Verification items for the finished model (mm, model axes). Face numbers are marked on the shaded views. A direction names the side the tool comes from. Give positions to 0.01 mm unless a question says otherwise; leave off trailing zeros. Order: outer loops, then holes, each group sorted by start corner. A loop starts at its lowest first (then second) coordinate and runs counter-clockwise, first axis right, second up. Notation, with made-up numbers: (49.25, 34) - (86.25, 34) arc R22 ccw to (86.25, 62) - close; hole circle Ø6 at (-5, -32). An arc over 180 degrees is marked (long way). Answer as a JSON object with one key per item and string values. Group by question number.
(1) Thickness scan on line 1 (X direction, y = 1.95, z = 0); line 2 (X direction, y = 5.5, z = 0); line 3 (Y direction, x = -5, z = 2.25). Record the ranges inside material, lowest first.
(2) Mould release check, pull along Z, two halves, no side actions. Record for the marked faces 6, 7 and 8: +Z half, -Z half, draft (parallel to the pull), parting line (faces both ways), or undercut.
(3) Access from +Z, -Z, +X, -X, +Y, -Y to the whole of each face (thin tool, end or side, straight path). Record for the marked faces 1, 2, 3, 4 and 5.
(4) Section check B-B (y = 5.75). Record the boundary of the cut face in (x, z).
(5) Section check C-C (z = 0.75). Record the boundary of the cut face in (x, y), then the cut area to 3 significant figures.
(6) Section check A-A (x = 2). Record the boundary of the cut face in (y, z).
(7) Depth check by flat-ended pin: pin 1 Ø5.5 at (x, z) = (2, 0) entering from +Y; pin 2 Ø2 at (x, y) = (-4.5, 11.5) entering from +Z; pin 3 Ø1.5 at (y, z) = (10, 1) entering from -X. Enter the tip coordinate at first touch or a pass-through.
(8) Section check D-D (x = -6.8). Record the boundary of the cut face in (y, z).
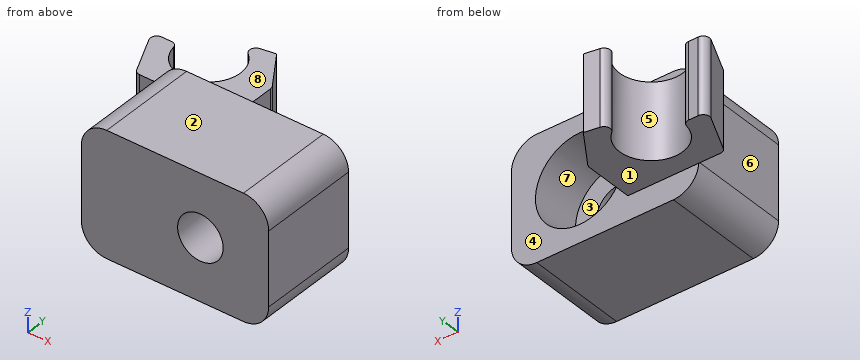
```python
from build123d import *

# Parameters (mm, degrees)
BOSS_EXTRUDE1_DEPTH      = 8
SKETCH2_R                = 3.5
CUT_EXTRUDE1_DEPTH       = 4
SKETCH3_R                = 1.8
CUT_EXTRUDE2_DEPTH       = 4
BOSS_EXTRUDE2_DEPTH      = 3
BOSS_EXTRUDE2_DEPTH_BACK = 3
FILLET1_R                = 0.5


with BuildPart() as part:
    # Sketch1 → Boss-Extrude1 (new body)
    with BuildSketch(Plane(origin=(0, 0, 0), x_dir=(1, 0, 0), z_dir=(0, 1, 0))):
        with BuildLine():
            Line((-5.4, -4.9), (5.4, -4.9))
            ThreePointArc((5.4, -4.9), (6.814213562, -4.314213562), (7.4, -2.9))
            Line((7.4, -2.9), (7.4, 2.9))
            ThreePointArc((7.4, 2.9), (6.814213562, 4.314213562), (5.4, 4.9))
            Line((5.4, 4.9), (-5.4, 4.9))
            ThreePointArc((-5.4, 4.9), (-6.814213562, 4.314213562), (-7.4, 2.9))
            Line((-7.4, 2.9), (-7.4, -2.9))
            ThreePointArc((-7.4, -2.9), (-6.814213562, -4.314213562), (-5.4, -4.9))
        make_face()
    extrude(amount=BOSS_EXTRUDE1_DEPTH)

    # Sketch2 → Cut-Extrude1 (cut)
    with BuildSketch(Plane(origin=(0, 8, 0), x_dir=(1, 0, 0), z_dir=(0, 1, 0))):
        with Locations(Location((2, 0, 0), (0, 0, 270))):
            Circle(SKETCH2_R)
    extrude(amount=-CUT_EXTRUDE1_DEPTH, mode=Mode.SUBTRACT)

    # Sketch3 → Cut-Extrude2 (cut)
    with BuildSketch(Plane(origin=(0, 4, 0), x_dir=(1, 0, 0), z_dir=(0, 1, 0))):
        with Locations(Location((2, 0, 0), (0, 0, 270))):
            Circle(SKETCH3_R)
    extrude(amount=-CUT_EXTRUDE2_DEPTH, mode=Mode.SUBTRACT)

    # Sketch4 → Boss-Extrude2 (add, two sides: drawn at the far end of the back side and taken through both)
    with BuildSketch(Plane.XY.offset(-BOSS_EXTRUDE2_DEPTH_BACK)):
        with BuildLine():
            ThreePointArc((-9.3, 12), (-5.032233047, 10.232233047), (-6.8, 14.5))
            Line((-6.8, 14.5), (-3.8, 15))
            Line((-3.8, 15), (-1.8, 12))
            Line((-1.8, 12), (-1.8, 8))
            Line((-1.8, 8), (-7.4, 8))
            Line((-7.4, 8), (-9.434769367, 8))
            Line((-9.434769367, 8), (-11.3, 12))
            Line((-11.3, 12), (-9.3, 12))
        make_face()
    extrude(amount=BOSS_EXTRUDE2_DEPTH + BOSS_EXTRUDE2_DEPTH_BACK)

    # Fillet1
    fillet1_edges = [part.edges().sort_by_distance(p)[0] for p in [
        (-9.3, 12, 0),
        (-6.8, 14.5, 0),
        (-1.8, 12, 0),
        (-9.434769367, 8, 0),
        (-11.3, 12, 0),
    ]]
    fillet(fillet1_edges, radius=FILLET1_R)


solid = part.part
```
Solutions:
{
 "1": {"line 1": "x = -7.4 to 0.2, 3.8 to 7.4", "line 2": "x = -7.4 to -1.5, 5.5 to 7.4", "line 3": "y = 0 to 10.27, 13.73 to 14.8"},
 "2": {"face 6": "draft", "face 7": "undercut", "face 8": "+Z half"},
 "3": {"face 1": "-Z, +X, -X, +Y", "face 2": "+Z, +X, -X, +Y, -Y", "face 3": "+Y", "face 4": "+X, +Y", "face 5": "+Z, -Z"},
 "4": {"outline": "(-7.4, -2.9) arc R2 ccw to (-5.4, -4.9) - (5.4, -4.9) arc R2 ccw to (7.4, -2.9) - (7.4, 2.9) arc R2 ccw to (5.4, 4.9) - (-5.4, 4.9) arc R2 ccw to (-7.4, 2.9) - close; hole circle Ø7 at (2, 0)"},
 "5": {"outline": "(-10.97, 11.29) - (-9.57, 8.29) arc R0.5 ccw to (-9.12, 8) - (-7.4, 8) - (-7.4, 0) - (0.36, 0) - (0.36, 4) - (-1.42, 4) - (-1.42, 8) - (-1.8, 8) - (-1.8, 11.85) arc R0.5 ccw to (-1.88, 12.13) - (-3.8, 15) - (-4.97, 14.8) arc R0.5 ccw to (-5.21, 13.93) arc R2.5 cw (long way) to (-9.27, 11.58) arc R0.5 ccw to (-9.76, 12) - (-10.52, 12) arc R0.5 ccw to start; (3.64, 0) - (7.4, 0) - (7.4, 8) - (5.42, 8) - (5.42, 4) - (3.64, 4) - close", "area": "108 mm2"},
 "6": {"outline": "(0, -4.9) - (8, -4.9) - (8, -3.5) - (4, -3.5) - (4, -1.8) - (0, -1.8) - close; (0, 1.8) - (4, 1.8) - (4, 3.5) - (8, 3.5) - (8, 4.9) - (0, 4.9) - close"},
 "7": {"pin 1": "stops at y = 4", "pin 2": "stops at z = 3", "pin 3": "stops at x = -10.72"},
 "8": {"outline": "(0, -4.33) - (8, -4.33) - (8, -3) - (9.5, -3) - (9.5, 3) - (8, 3) - (8, 4.33) - (0, 4.33) - close"}
}
